Part model, mm, in its own coordinate system. Face numbers are marked on the shaded views. A direction names the side the tool comes from. Round coordinates to 2 decimals unless told otherwise and drop trailing zeros. Order: outer loops, then holes, each group sorted by start corner. A loop starts at its lowest first (then second) coordinate and runs counter-clockwise, first axis right, second up. Notation, with made-up numbers: (36, 34.5) - (88, 34.5) arc R21 ccw to (88, 39.5) - close; hole circle Ø11 at (44, 51.25). An arc over 180 degrees is marked (long way). Answer as a JSON object with one key per item and string values.
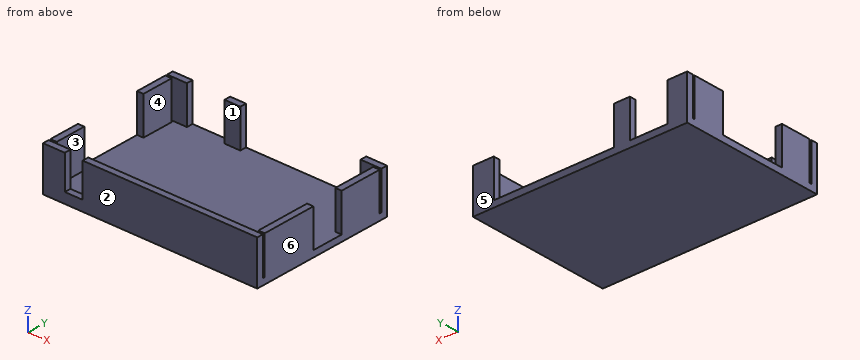
```python
from build123d import *

# Parameters (mm, degrees)
SKETCH1_W           = 108.2
SKETCH1_H           = 73.5
BOSS_EXTRUDE2_DEPTH = 3.2
SKETCH2_W           = 108.2
SKETCH2_H           = 73.5
SKETCH2_W_2         = 101.8
SKETCH2_H_2         = 67.1
BOSS_EXTRUDE3_DEPTH = 19
SKETCH3_W           = 3.2
SKETCH3_H           = 1
CUT_EXTRUDE1_DEPTH  = 19
SKETCH4_W           = 3.2
SKETCH4_H           = 33.5
CUT_EXTRUDE2_DEPTH  = 19
SKETCH5_W           = 19
SKETCH5_H           = 3.2
SKETCH5_W_2         = 60.7
CUT_EXTRUDE3_DEPTH  = 19
SKETCH6_W           = 3.2
SKETCH6_H           = 16
CUT_EXTRUDE4_DEPTH  = 19
SKETCH7_W           = 9
SKETCH7_H           = 3.2
CUT_EXTRUDE5_DEPTH  = 17


with BuildPart() as part:
    # Sketch1 → Boss-Extrude2 (new body)
    with BuildSketch(Plane.XY):
        with Locations((54.1, 36.75)):
            Rectangle(SKETCH1_W, SKETCH1_H)
    extrude(amount=BOSS_EXTRUDE2_DEPTH)

    # Sketch2 → Boss-Extrude3 (add)
    with BuildSketch(Plane.XY.offset(3.2)):
        with Locations((54.1, 36.75)):
            Rectangle(SKETCH2_W, SKETCH2_H)
        with Locations((54.1, 36.75)):
            Rectangle(SKETCH2_W_2, SKETCH2_H_2, mode=Mode.SUBTRACT)
    extrude(amount=BOSS_EXTRUDE3_DEPTH)

    # Sketch3 → Cut-Extrude1 (cut)
    with BuildSketch(Plane.XY.offset(22.2)):
        with Locations((1.6, 69.8)):
            Rectangle(SKETCH3_W, SKETCH3_H)
        with Locations((106.6, 69.8)):
            Rectangle(SKETCH3_W, SKETCH3_H)
        with Locations((106.6, 3.7)):
            Rectangle(SKETCH3_W, SKETCH3_H)
        with Locations((1.6, 3.7)):
            Rectangle(SKETCH3_W, SKETCH3_H)
    extrude(amount=-CUT_EXTRUDE1_DEPTH, mode=Mode.SUBTRACT)

    # Sketch4 → Cut-Extrude2 (cut)
    with BuildSketch(Plane.XY.offset(22.2)):
        with Locations((1.6, 36.55)):
            Rectangle(SKETCH4_W, SKETCH4_H)
    extrude(amount=-CUT_EXTRUDE2_DEPTH, mode=Mode.SUBTRACT)

    # Sketch5 → Cut-Extrude3 (cut)
    with BuildSketch(Plane.XY.offset(22.2)):
        with Locations((19.5, 71.9)):
            Rectangle(SKETCH5_W, SKETCH5_H)
        with Locations((67.35, 71.9)):
            Rectangle(SKETCH5_W_2, SKETCH5_H)
    extrude(amount=-CUT_EXTRUDE3_DEPTH, mode=Mode.SUBTRACT)

    # Sketch6 → Cut-Extrude4 (cut)
    with BuildSketch(Plane.XY.offset(22.2)):
        with Locations((106.6, 39.8)):
            Rectangle(SKETCH6_W, SKETCH6_H)
    extrude(amount=-CUT_EXTRUDE4_DEPTH, mode=Mode.SUBTRACT)

    # Sketch7 → Cut-Extrude5 (cut)
    with BuildSketch(Plane.XY.offset(22.2)):
        with Locations((15.5, 1.6)):
            Rectangle(SKETCH7_W, SKETCH7_H)
    extrude(amount=-CUT_EXTRUDE5_DEPTH, mode=Mode.SUBTRACT)


solid = part.part
```
Item 1: Probe L1, parallel to X at y = 53.5, z = 18.75; L2, parallel to Y at x = 100, z = 13.75; L3, parallel to Z at x = 75, y = 47.5. List the from-to ranges inside material, lowest first. Write a range as from..to.
Taken from the geometry:
{"L1": "0..3.2, 105..108.2", "L2": "0..3.2, 70.3..73.5", "L3": "0..3.2"}
Item 2: Two-plate mould, pull along Y, no slides. Class the marked faces 4, 5 and 6: pulls with the +Y half, pulls with the -Y half, needs draft (parallel to the pull), parting line crosses it, or undercut.
Taken from the geometry:
{"face 4": "undercut", "face 5": "pulls with the +Y half", "face 6": "needs draft"}
Item 3: Tool access for the marked faces 1, 2 and 3: list every direction of +Z, -Z, +X, -X, +Y, -Y with a clear straight run to the whole face (end or side of a thin tool).
Taken from the geometry:
{"face 1": "+Z, +X, -X", "face 2": "+Z, -Z, +X, -X, -Y", "face 3": "+Z"}
Item 4: Cut at C-C (z = 10.75). State how many separate pieces and enclosed holes the cut face has, plus the area to 3 significant figures.
Taken from the geometry:
{"separate pieces": "9", "enclosed holes": "0", "area": "667 mm2"}
Item 5: Cut at A-A (y = 68). Write the cut outline in (x, z), plus the area to 3 significant figures.
Taken from the geometry:
{"outline": "(0, 0) - (108.2, 0) - (108.2, 22.2) - (105, 22.2) - (105, 3.2) - (3.2, 3.2) - (3.2, 22.2) - (0, 22.2) - close", "area": "468 mm2"}
Item 6: Drop flat-ended pins along their axis: P1, Ø1.5, axis at y = 49, z = 16.5, coming from the -X side; P2, Ø3, axis at x = 72.5, y = 9, coming from the +Z side; P3, Ø3.5, axis at x = 14, y = 1.5, coming from the +Z side. Give the stop position or say it passes through.
Taken from the geometry:
{"P1": "x = 105", "P2": "z = 3.2", "P3": "z = 5.2"}
Item 7: Cut at B-B (x = 66). Write the cut outline in (y, z), plus the area to 3 significant figures.
Taken from the geometry:
{"outline": "(0, 0) - (73.5, 0) - (73.5, 3.2) - (3.2, 3.2) - (3.2, 22.2) - (0, 22.2) - close", "area": "296 mm2"}
Item 8: Cut at D-D (y = 49). Write the cut outline in (x, z), plus the area to 3 significant figures.
Taken from the geometry:
{"outline": "(0, 0) - (108.2, 0) - (108.2, 22.2) - (105, 22.2) - (105, 3.2) - (0, 3.2) - close", "area": "407 mm2"}
